Input: dimensioned drawing with shaded views. Units: mm. Origin: part minimum x, y, z. Give positions to 0.01 mm unless a question says otherwise; leave off trailing zeros. Loops run counter-clockwise (first coordinate to the right, second up) from the corner with the lowest first, then second, coordinate; pieces in that order, holes last.
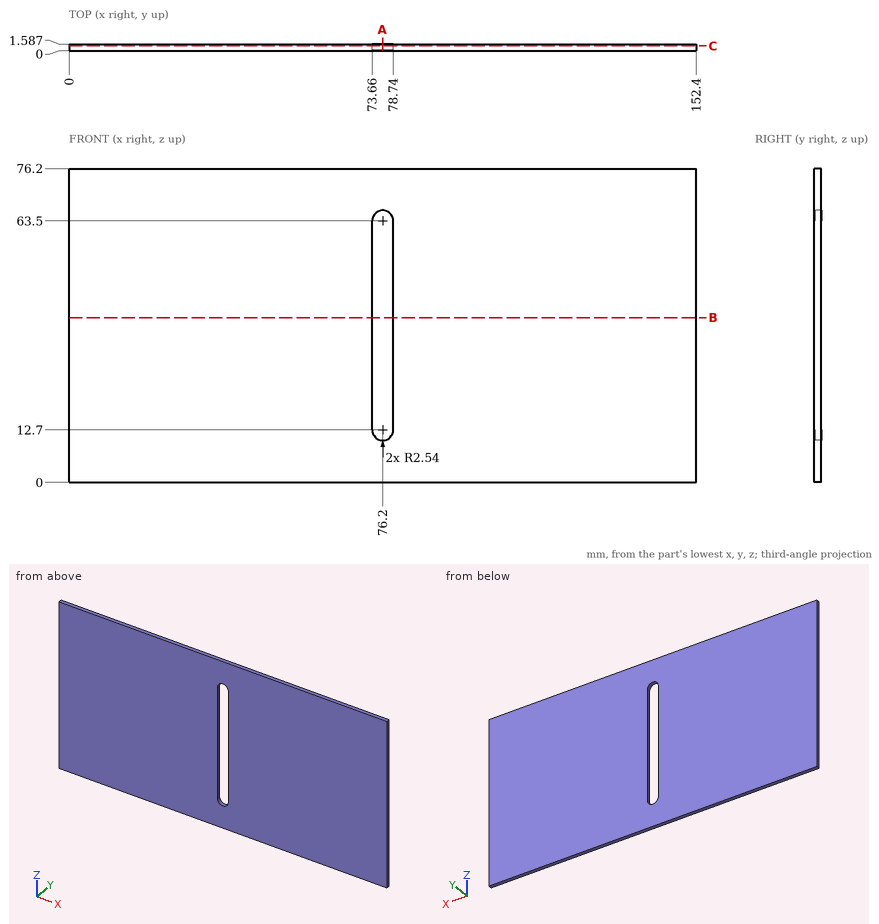
(1) Section C-C, the plane y = 1.15. Return the cut outline in (x, z), then the cut area to 3 significant figures.
A:
outline: (0, 0) - (152.4, 0) - (152.4, 76.2) - (0, 76.2) - close; hole (73.66, 12.7) arc R2.54 ccw to (78.74, 12.7) - (78.74, 63.5) arc R2.54 ccw to (73.66, 63.5) - close
area: 11,300 mm2
(2) First-contact query: pin 1 (10 mm diameter, centred on x = 77, z = 15.5, fed in from -Y). Flat tip, straight axial feed; report the tip coordinate or a pass-through.
A:
pin 1: stops at y = 0
(3) Section B-B, the plane z = 40. Return the cut outline in (x, y), then the cut area to 3 significant figures.
A:
outline: (0, 0) - (73.66, 0) - (73.66, 1.59) - (0, 1.59) - close; (78.74, 0) - (152.4, 0) - (152.4, 1.59) - (78.74, 1.59) - close
area: 234 mm2
(4) Ray query, line 1 along X through (y, z) = (0.8, 30); line 2 along Z through (x, y) = (76.5, 0.35). Return the intervals inside material, ascending.
A:
line 1: x = 0 to 73.66, 78.74 to 152.4
line 2: z = 0 to 10.18, 66.02 to 76.2
(5) Section A-A, the plane x = 76.2. Return the cut outline in (y, z).
A:
outline: (0, 0) - (1.59, 0) - (1.59, 10.16) - (0, 10.16) - close; (0, 66.04) - (1.59, 66.04) - (1.59, 76.2) - (0, 76.2) - close
